```python
from build123d import *

# Parameters (mm, degrees)
SKETCH1_W                                      = 69.85
SKETCH1_H                                      = 101.6
BOSS_EXTRUDE1_DEPTH                            = 9.525
F_1_4_20_TAPPED_HOLE1_D                        = 5.1054
F_1_4_20_TAPPED_HOLE1_DEPTH                    = 19.05
F_1_4_20_TAPPED_HOLE1_TIP                      = 1.533816902
F_18_0_18_DIAMETER_HOLE1_D                     = 18
CBORE_FOR_M5_HEX_HEAD_BOLT1_D                  = 5.5
CBORE_FOR_M5_HEX_HEAD_BOLT1_CBORE_D            = 12.24
CBORE_FOR_M5_HEX_HEAD_BOLT1_CBORE_DEPTH        = 3.58
CBORE_FOR_4_SOCKET_HEAD_CAP_SCREW1_D           = 3.2639
CBORE_FOR_4_SOCKET_HEAD_CAP_SCREW1_CBORE_D     = 5.55752
CBORE_FOR_4_SOCKET_HEAD_CAP_SCREW1_CBORE_DEPTH = 2.8448
F_10_CLEARANCE_SLOT1_DEPTH                     = 9.525
SKETCH23_W                                     = 3.175
SKETCH23_H                                     = 101.6
BOSS_EXTRUDE2_DEPTH                            = 9.525
CUT_EXTRUDE2_DEPTH                             = 126.482812568


# Read off the part's stored shape, not the designer's step: #10 Clearance Slot1
with BuildPart() as part:
    # Sketch1 → Boss-Extrude1 (new body)
    with BuildSketch(Plane(origin=(0, 0, 0), x_dir=(1, 0, 0), z_dir=(0, 1, 0))):
        with Locations((34.925, 50.8)):
            Rectangle(SKETCH1_W, SKETCH1_H)
    extrude(amount=BOSS_EXTRUDE1_DEPTH)

    # 1/4-20 Tapped Hole1
    with Locations(Plane.XY):
        with Locations((8.73125, 4.7625), (61.11875, 4.7625), (34.925, 4.7625)):
            Hole(F_1_4_20_TAPPED_HOLE1_D / 2, depth=F_1_4_20_TAPPED_HOLE1_DEPTH)
            with Locations((0, 0, -(F_1_4_20_TAPPED_HOLE1_DEPTH + F_1_4_20_TAPPED_HOLE1_TIP / 2))):  # 118° drill point
                Cone(0, F_1_4_20_TAPPED_HOLE1_D / 2, F_1_4_20_TAPPED_HOLE1_TIP, mode=Mode.SUBTRACT)

    # Ø18.0 (18) Diameter Hole1 (through all)
    with Locations(Plane(origin=(0, 9.525, 0), x_dir=(1, 0, 0), z_dir=(0, 1, 0))):
        with Locations((50.200768572, 42.808816902)):
            Hole(F_18_0_18_DIAMETER_HOLE1_D / 2)

    # CBORE for M5 Hex Head Bolt1 (through all)
    with Locations(Plane(origin=(0, 9.525, 0), x_dir=(1, 0, 0), z_dir=(0, 1, 0))):
        with Locations((52.379662144, 67.713684392), (48.021875, 17.903949412)):
            CounterBoreHole(CBORE_FOR_M5_HEX_HEAD_BOLT1_D / 2, CBORE_FOR_M5_HEX_HEAD_BOLT1_CBORE_D / 2, CBORE_FOR_M5_HEX_HEAD_BOLT1_CBORE_DEPTH)

    # CBORE for #4 Socket Head Cap Screw1 (through all)
    with Locations(Plane(origin=(0, 0, 0), x_dir=(-1, 0, 0), z_dir=(0, -1, 0))):
        with Locations((-25.814021811, 60.200257539), (-66.075768572, 55.508816902)):
            CounterBoreHole(CBORE_FOR_4_SOCKET_HEAD_CAP_SCREW1_D / 2, CBORE_FOR_4_SOCKET_HEAD_CAP_SCREW1_CBORE_D / 2, CBORE_FOR_4_SOCKET_HEAD_CAP_SCREW1_CBORE_DEPTH)

    # #10 Clearance Slot1 outline → #10 Clearance Slot1 (cut)
    with BuildSketch(Plane(origin=(0, 0, 0), x_dir=(1, 0, 0), z_dir=(0, 1, 0))):
        with BuildLine():
            Line((18.030825, 18.474656367), (25.625425, 18.474656367))
            ThreePointArc((25.625425, 18.474656367), (28.178125, 21.027356367), (25.625425, 23.580056367))
            Line((25.625425, 23.580056367), (18.030825, 23.580056367))
            ThreePointArc((18.030825, 23.580056367), (15.478125, 21.027356367), (18.030825, 18.474656367))
        make_face()
    extrude(amount=F_10_CLEARANCE_SLOT1_DEPTH, mode=Mode.SUBTRACT)

    # Sketch23 → Boss-Extrude2 (add)
    with BuildSketch(Plane(origin=(0, 0, 0), x_dir=(1, 0, 0), z_dir=(0, 1, 0))):
        with Locations((71.4375, 50.8)):
            Rectangle(SKETCH23_W, SKETCH23_H)
        with Locations((-1.5875, 50.8)):
            Rectangle(SKETCH23_W, SKETCH23_H)
    extrude(amount=BOSS_EXTRUDE2_DEPTH)

    # Sketch24 → Cut-Extrude2 (cut, through all)
    with BuildSketch(Plane(origin=(0, 0, 0), x_dir=(1, 0, 0), z_dir=(0, 1, 0))):
        with BuildLine():
            ThreePointArc((60.086847532, 73.833684392), (69.661188781, 59.594122619), (73.025, 42.768014811))
            Line((73.025, 42.768014811), (73.025, 101.6))
            Line((73.025, 101.6), (-3.175, 101.6))
            Line((-3.175, 101.6), (-3.175, 12.7))
            ThreePointArc((-3.175, 12.7), (-2.45000516, 18.323895492), (-0.322426517, 23.580056367))
            Line((-0.322426517, 23.580056367), (22.97958653, 64.963684392))
            ThreePointArc((22.97958653, 64.963684392), (31.651165616, 73.776549238), (43.584990358, 77.008684392))
            Line((43.584990358, 77.008684392), (52.379662144, 77.008684392))
            ThreePointArc((52.379662144, 77.008684392), (56.547435278, 76.183844834), (60.086847532, 73.833684392))
        make_face()
    extrude(amount=CUT_EXTRUDE2_DEPTH, mode=Mode.SUBTRACT)


solid = part.part
```
Here's how the part is built. I have some questions about the finished solid (model axes, mm). A direction names the side the tool comes from. Coordinates: 2 decimals unless noted, no trailing zeros. Order: outer loops, then holes, each group sorted by start corner. A loop starts at its lowest first (then second) coordinate and runs counter-clockwise, first axis right, second up. Notation, with made-up numbers: (26.25, -37) -> (40.25, -37) arc R34 ccw to (40.25, -2) -> close; hole circle Ø7 at (85, 48.25). An arc over 180 degrees is marked (long way). Return JSON: item names as keys, results as strings.
1) If we section it at A-A on y = 1: List the corners of the cut face in (x, z) for me (3 decimals), plus the area to 3 significant figures.
Conclusion:
{"outline": "(-3.175, -12.7) arc R22.175 ccw to (-0.322, -23.58) -> (22.98, -64.964) arc R23.647 ccw to (43.585, -77.009) -> (52.38, -77.009) arc R10.942 ccw to (60.087, -73.834) arc R43.765 ccw to (73.025, -42.768) -> (73.025, 0) -> (-3.175, 0) -> close; hole (18.031, -23.58) -> (25.625, -23.58) arc R2.553 ccw to (25.625, -18.475) -> (18.031, -18.475) arc R2.553 ccw to start; hole circle Ø5.558 at (25.814, -60.2); hole circle Ø18 at (50.201, -42.809); hole circle Ø5.5 at (48.022, -17.904); hole circle Ø5.5 at (52.38, -67.714); hole circle Ø5.558 at (66.076, -55.509)", "area": "4,290 mm²"}
2) If we section it at B-B on z = -45.5: List the corners of the cut face in (x, y) for me (3 decimals), plus the area to 3 significant figures.
Conclusion:
{"outline": "(12.02, 0) -> (41.613, 0) -> (41.613, 9.525) -> (12.02, 9.525) -> close; (58.789, 0) -> (72.94, 0) -> (72.94, 9.525) -> (58.789, 9.525) -> close", "area": "417 mm²"}
3) If we section it at C-C on z = -9.5: List the corners of the cut face in (x, y) for me (1 decimal).
Conclusion:
{"outline": "(-3.2, 0) -> (73, 0) -> (73, 9.5) -> (-3.2, 9.5) -> close; hole circle Ø5.1 at (8.7, 4.8); hole circle Ø5.1 at (34.9, 4.8); hole circle Ø5.1 at (61.1, 4.8)"}
4) Thinking about a two-plate mould opening in Y: for faces 1 (the conical face through (35.348, 4.896, -20.317)), 2 (the flat face through (34, 9.525, -30)), 3 (the flat face through (73.025, 5, -21)), which applies, +Y half, -Y half, draft (parallel to the pull), parting line (faces both ways), or undercut?
Conclusion:
{"face 1": "undercut", "face 2": "+Y half", "face 3": "draft"}
5) On a 3-axis mill with a long thin cutter (end or side, diameter ignored), from which of +Z, -Z, +X, -X, +Y, -Y can I reach the whole of each face in a straight line? I mean faces 4 (the flat face through (24, 2.845, -60)), 5 (the cylindrical face through (15.48, 4.7, -21.08)), 6 (the cylindrical face through (69.568, 4.696, -59.817)), 7 (the cylindrical face through (58.684, 5.529, -9.658)), 8 (the cylindrical face through (47.225, 7.76, -23.972)). Say none if no direction works.
Conclusion:
{"face 4": "-Y", "face 5": "+Y, -Y", "face 6": "-Z, +X, +Y, -Y", "face 7": "+Z", "face 8": "+Y"}
6) If I drill on probe 1 along X at (y, z) = (2, -58); probe 2 along Z at (x, y) = (52.5, 7.5); probe 3 along X at (y, z) = (4.5, -18) (3 decimals), over which ranges is the centre line in solid material (lowest first)?
Conclusion:
{"probe 1": "x = 19.06 to 24.12, 27.51 to 64.84, 67.31 to 70.29", "probe 2": "z = -77.01 to -73.83, -61.59 to -51.51, -34.11 to -22.08, -13.73 to 0", "probe 3": "x = -2.532 to 6.192, 11.27 to 32.386, 37.464 to 45.274, 50.77 to 58.58, 63.658 to 73.025"}
7) I'm going to push flat-ended pins straight in: P1, Ø3, axis at x = 34.92, y = 4.76, coming from the +Z side; P2, Ø1.5, axis at y = 4.5, z = -52.5, coming from the +X side; P3, Ø4, axis at x = 26.5, y = 2.5, coming from the -Z side. Where does each tip first touch, or does it pass through?
Conclusion:
{"P1": "stops at z = -19.68", "P2": "stops at x = 72.09", "P3": "stops at z = -71.57"}
